Print and shaded views of the part. All mm, measured from the part's lowest x, y and z. Round coordinates to 2 decimals unless told otherwise and drop trailing zeros. Order: outer loops, then holes, each group sorted by start corner. A loop starts at its lowest first (then second) coordinate and runs counter-clockwise, first axis right, second up. Notation, with made-up numbers: (-14, -29) - (37, -29) arc R6 cw to (37, -20) - close; hole circle Ø10 at (-23.5, 5). An arc over 180 degrees is marked (long way). Return JSON: item names as keys, results as strings. Group by question number.
Item 1: Saw through at D-D on x = 14.5. List the corners of the cut face in (y, z), and give its area (3 significant figures).
Item 2: Saw through at C-C on y = 10.5. List the corners of the cut face in (x, z).
Item 3: Saw through at B-B on z = 1.05. State how many separate pieces and enclosed holes the cut face has, and give its area (3 significant figures).
Item 4: Drop flat-ended pins along their axis: pin 1 (2 mm diameter, centred on y = 10, z = 3, fed in from -X); pin 2 (1.2 mm diameter, centred on x = 57.5, z = 2, fed in from -Y); pin 3 (2 mm diameter, centred on y = 10.5, z = 1, fed in from +X). Give the stop position or say it passes through.
Item 5: Saw through at A-A on x = 55. List the corners of the cut face in (y, z), and give its area (3 significant figures).
Item 6: Probe probe 1 along X at (y, z) = (47, 1.9); probe 2 along Y at (x, z) = (7.5, 2.25); probe 3 along X at (y, z) = (12, 2.25). List the from-to ranges inside material, lowest first.
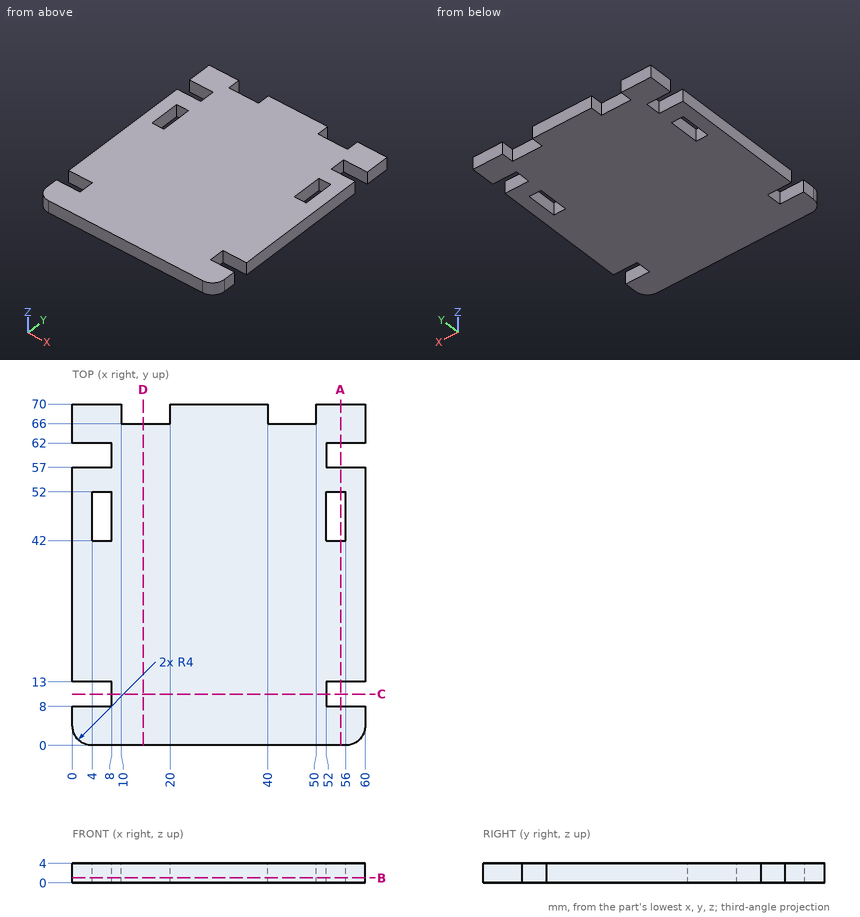
Filled in:
{
 "1": {"outline": "(0, 0) - (66, 0) - (66, 4) - (0, 4) - close", "area": "264 mm^2"},
 "2": {"outline": "(8, 0) - (52, 0) - (52, 4) - (8, 4) - close"},
 "3": {"separate pieces": "1", "enclosed holes": "2", "area": "3,870 mm^2"},
 "4": {"pin 1": "stops at x = 8", "pin 2": "stops at y = 0.1", "pin 3": "stops at x = 52"},
 "5": {"outline": "(0, 0) - (8, 0) - (8, 4) - (0, 4) - close; (13, 0) - (42, 0) - (42, 4) - (13, 4) - close; (52, 0) - (57, 0) - (57, 4) - (52, 4) - close; (62, 0) - (70, 0) - (70, 4) - (62, 4) - close", "area": "200 mm^2"},
 "6": {"probe 1": "x = 0 to 4, 8 to 52, 56 to 60", "probe 2": "y = 0 to 8, 13 to 42, 52 to 57, 62 to 70", "probe 3": "x = 8 to 52"}
}
